```python
from build123d import *

# Parameters (mm, degrees)
SKETCH1_W               = 30
SKETCH1_H               = 30
BOSS_EXTRUDE1_DEPTH     = 5
SKETCH4_R               = 10
BOSS_EXTRUDE2_DEPTH     = 10
CUT_EXTRUDE3_DEPTH      = 26.980762114
CUT_EXTRUDE3_DEPTH_BACK = 26.980762114
SKETCH5_R               = 2
SKETCH6_R               = 4.5
SKETCH6_R_2             = 3.5
CUT_EXTRUDE4_DEPTH      = 7
CHAMFER1_SIZE           = 10
CHAMFER1_SIZE_2         = 4.040262258
CUT_EXTRUDE5_DEPTH      = 24.452078799
CUT_EXTRUDE5_DEPTH_BACK = 24.452078799
SKETCH8_R               = 1.5
SKETCH9_R               = 2.5
CUT_EXTRUDE6_DEPTH      = 2
FILLET1_R               = 5
CHAMFER2_SIZE           = 7
CHAMFER2_SIZE2          = 4.901452767


with BuildPart() as part:
    # Sketch1 → Boss-Extrude1 (new body)
    with BuildSketch(Plane(origin=(0, 0, 0), x_dir=(1, 0, 0), z_dir=(0, 1, 0))):
        Rectangle(SKETCH1_W, SKETCH1_H)
    extrude(amount=BOSS_EXTRUDE1_DEPTH)

    # Sketch4 → Boss-Extrude2 (add)
    with BuildSketch(Plane(origin=(0, 5, 0), x_dir=(1, 0, 0), z_dir=(0, 1, 0))):
        with Locations(Location((0, 0, 0), (0, 0, 270))):
            Circle(SKETCH4_R)
    extrude(amount=BOSS_EXTRUDE2_DEPTH)

    # Sketch5 → Cut-Extrude3 (cut, two sides: drawn at the far end of the back side and taken through both)
    with BuildSketch(Plane(origin=(0, 15, 0), x_dir=(1, 0, 0), z_dir=(0, 1, 0)).offset(-CUT_EXTRUDE3_DEPTH_BACK)):
        with Locations(Location((0, 0, 0), (0, 0, 270))):
            Circle(SKETCH5_R)
    extrude(amount=CUT_EXTRUDE3_DEPTH + CUT_EXTRUDE3_DEPTH_BACK, mode=Mode.SUBTRACT)

    # Sketch6 → Cut-Extrude4 (cut)
    with BuildSketch(Plane(origin=(0, 15, 0), x_dir=(1, 0, 0), z_dir=(0, 1, 0))):
        with Locations(Location((0, 0, 0), (0, 0, 270))):
            Circle(SKETCH6_R)
        with Locations(Location((0, 0, 0), (0, 0, 270))):
            Circle(SKETCH6_R_2, mode=Mode.SUBTRACT)
    extrude(amount=-CUT_EXTRUDE4_DEPTH, mode=Mode.SUBTRACT)

    # Chamfer1
    # the kernel refuses this chamfer: 10, 4.040262258 mm, written as the material it takes off along each edge
    with BuildSketch(Plane(origin=(0, 15, 0), x_dir=(0, 0, 1), z_dir=(-1, 0, 0))) as chamfer1_piece_1_section:
        Polygon((10, -CHAMFER1_SIZE), (10 - CHAMFER1_SIZE_2, 0), (10, 0), align=None)
    chamfer1_piece_1 = revolve(axis=Axis((0, 15, 0), (0, 1, 0)), mode=Mode.PRIVATE)
    chamfer1_piece_1 = split(chamfer1_piece_1, bisect_by=Plane(origin=(0, 5, -8.005876014), z_dir=(0, 1, 0)), keep=Keep.TOP, mode=Mode.PRIVATE)
    add(chamfer1_piece_1, mode=Mode.SUBTRACT)

    # Sketch8 → Cut-Extrude5 (cut, two sides: drawn at the far end of the back side and taken through both)
    with BuildSketch(Plane(origin=(0, 5, 0), x_dir=(1, 0, 0), z_dir=(0, 1, 0)).offset(-CUT_EXTRUDE5_DEPTH_BACK)):
        with Locations(Location((10.5, 10.5, 0), (0, 0, 270))):
            Circle(SKETCH8_R)
        with Locations(Location((10.5, -10.5, 0), (0, 0, 270))):
            Circle(SKETCH8_R)
        with Locations(Location((-10.5, -10.5, 0), (0, 0, 270))):
            Circle(SKETCH8_R)
        with Locations(Location((-10.5, 10.5, 0), (0, 0, 270))):
            Circle(SKETCH8_R)
    extrude(amount=CUT_EXTRUDE5_DEPTH + CUT_EXTRUDE5_DEPTH_BACK, mode=Mode.SUBTRACT)

    # Sketch9 → Cut-Extrude6 (cut)
    with BuildSketch(Plane(origin=(0, 5, 0), x_dir=(1, 0, 0), z_dir=(0, 1, 0))):
        with Locations(Location((-10.5, 10.5, 0), (0, 0, 270))):
            Circle(SKETCH9_R)
        with Locations(Location((10.5, 10.5, 0), (0, 0, 270))):
            Circle(SKETCH9_R)
        with Locations(Location((10.5, -10.5, 0), (0, 0, 270))):
            Circle(SKETCH9_R)
        with Locations(Location((-10.5, -10.5, 0), (0, 0, 270))):
            Circle(SKETCH9_R)
    extrude(amount=-CUT_EXTRUDE6_DEPTH, mode=Mode.SUBTRACT)

    # Fillet1
    fillet1_edges = [part.edges().sort_by_distance(p)[0] for p in [
        (15, 2.5, 15),
        (-15, 2.5, 15),
        (-15, 2.5, -15),
        (15, 2.5, -15),
    ]]
    fillet(fillet1_edges, radius=FILLET1_R)

    # Chamfer2
    chamfer2_edges = [part.edges().sort_by_distance(p)[0] for p in [
        (0, 0, -2),
    ]]
    chamfer2_side = [part.faces().sort_by_distance(p)[0] for p in [
        (0, 7.5, -2),
    ]]
    chamfer(chamfer2_edges, length=CHAMFER2_SIZE, length2=CHAMFER2_SIZE2, reference=chamfer2_side[0])


solid = part.part
```
The model under review builds one solid part; all positions refer to its coordinate system, in mm. A direction names the side the tool comes from. Give positions to 0.01 mm unless a question says otherwise; leave off trailing zeros. Write each loop counter-clockwise with the first axis right and the second up, starting at its lowest first coordinate (ties: lowest second). Pieces come first, ordered by that corner, then holes. Notation, with made-up numbers: (-29, -25.5) -> (4, -25.5) arc R21 cw to (4, 0.5) -> close; hole circle Ø3 at (-37.75, 12). An arc over 180 degrees is marked (long way). Put each result on its own line as item: value.
(1) For pin 1 Ø4 at (x, z) = (9.5, -9.5) entering from +Y; pin 2 Ø1.5 at (x, z) = (-9.5, 10.5) entering from +Y; pin 3 Ø3 at (x, y) = (5.5, 11) entering from -Z, all flat-tipped, find the tip position at first contact; note any pin that passes through.
Results are:
pin 1: y = 5
pin 2: y = 3
pin 3: z = -6.67
(2) The part is to be moulded in two halves that separate along X. For faces 1 (the cylindrical face through (8.06, 4.01, -11.04)), 2 (the cylindrical face through (13, 3, -14)), 3 (the flat face through (6.5, 0, 3.1)), say which applies: pulls with the +X half, pulls with the -X half, needs draft (parallel to the pull), parting line crosses it, or undercut.
Results are:
face 1: undercut
face 2: pulls with the +X half
face 3: needs draft
(3) We need section C-C, the plane z = -10.5. Give the boundary of the cut face in (x, y).
Results are:
outline: (-14.97, 0) -> (-12, 0) -> (-12, 3) -> (-13, 3) -> (-13, 5) -> (-14.97, 5) -> close; (-9, 0) -> (9, 0) -> (9, 3) -> (8, 3) -> (8, 5) -> (-8, 5) -> (-8, 3) -> (-9, 3) -> close; (12, 0) -> (14.97, 0) -> (14.97, 5) -> (13, 5) -> (13, 3) -> (12, 3) -> close
(4) Tool access review of faces 4 (the flat face through (9, 3, 12)), 5 (the cylindrical face through (10.57, 1.48, -12)): name each direction out of +Z, -Z, +X, -X, +Y, -Y from which nothing blocks a thin tool from reaching the whole face with its end or side.
Results are:
face 4: +Y
face 5: +Y, -Y
(5) We need section D-D, the plane y = 2.5. Give the boundary of the cut face in (x, z).
Results are:
outline: (-15, -10) arc R5 ccw to (-10, -15) -> (10, -15) arc R5 ccw to (15, -10) -> (15, 10) arc R5 ccw to (10, 15) -> (-10, 15) arc R5 ccw to (-15, 10) -> close; hole circle Ø3 at (-10.5, -10.5); hole circle Ø3 at (-10.5, 10.5); hole circle Ø10.3 at (0, 0); hole circle Ø3 at (10.5, -10.5); hole circle Ø3 at (10.5, 10.5)
(6) To check wall thickness, follow probe 1 along X at (y, z) = (0.75, -10.5); probe 2 along X at (y, z) = (12.75, 0); probe 3 along Z at (x, y) = (-2.5, 9). State the ranges of each line that lie inside material, in increasing order. Write a range as from..to.
Results are:
probe 1: -14.97..-12, -9..9, 12..14.97
probe 2: -6.87..-4.5, -3.5..-2, 2..3.5, 4.5..6.87
probe 3: -8..-3.74, -2.45..2.45, 3.74..8
(7) We need section A-A, the plane x = 0. Give the boundary of the cut face in (y, z).
Results are:
outline: (0, -15) -> (5, -15) -> (5, -10) -> (15, -5.96) -> (15, -4.5) -> (8, -4.5) -> (8, -3.5) -> (15, -3.5) -> (15, -2) -> (7, -2) -> (0, -6.9) -> close; (0, 6.9) -> (7, 2) -> (15, 2) -> (15, 3.5) -> (8, 3.5) -> (8, 4.5) -> (15, 4.5) -> (15, 5.96) -> (5, 10) -> (5, 15) -> (0, 15) -> close
(8) We need section B-B, the plane z = 0. Give the boundary of the cut face in (x, y).
Results are:
outline: (-15, 0) -> (-6.9, 0) -> (-2, 7) -> (-2, 15) -> (-3.5, 15) -> (-3.5, 8) -> (-4.5, 8) -> (-4.5, 15) -> (-5.96, 15) -> (-10, 5) -> (-15, 5) -> close; (2, 7) -> (6.9, 0) -> (15, 0) -> (15, 5) -> (10, 5) -> (5.96, 15) -> (4.5, 15) -> (4.5, 8) -> (3.5, 8) -> (3.5, 15) -> (2, 15) -> close
